Read the model definition and answer for the solid it produces. Units are mm, in the model's axes. Round coordinates to 2 decimals unless told otherwise and drop trailing zeros. Order: outer loops, then holes, each group sorted by start corner. A loop starts at its lowest first (then second) coordinate and runs counter-clockwise, first axis right, second up.
from build123d import *

# Parameters (mm, degrees)
SKETCH1_R      = 3
EXTRUDE4_DEPTH = 10
EXTRUDE5_DEPTH = 50


with BuildPart() as part:
    # Sketch1 → Extrude4 (new body)
    with BuildSketch(Plane.XY):
        with BuildLine():
            Line((-20, 13.266499161), (-20, -13.266499161))
            ThreePointArc((-20, -13.266499161), (0, -24), (20, -13.266499161))
            Line((20, -13.266499161), (20, 13.266499161))
            ThreePointArc((20, 13.266499161), (0, 24), (-20, 13.266499161))
        make_face()
        with BuildLine():
            ThreePointArc((-9.899494937, 9.899494937), (-5.357568053, 12.934313455), (0, 14))
            ThreePointArc((0, 14), (5.357568053, 12.934313455), (9.899494937, 9.899494937))
            ThreePointArc((9.899494937, 9.899494937), (14, 0), (9.899494937, -9.899494937))
            ThreePointArc((9.899494937, -9.899494937), (5.357568053, -12.934313455), (0, -14))
            ThreePointArc((0, -14), (-5.357568053, -12.934313455), (-9.899494937, -9.899494937))
            ThreePointArc((-9.899494937, -9.899494937), (-14, 0), (-9.899494937, 9.899494937))
        make_face(mode=Mode.SUBTRACT)
        with Locations((-13.435028843, 13.435028843)):
            Circle(SKETCH1_R, mode=Mode.SUBTRACT)
        with Locations((0, 19)):
            Circle(SKETCH1_R, mode=Mode.SUBTRACT)
        with Locations((13.435028843, 13.435028843)):
            Circle(SKETCH1_R, mode=Mode.SUBTRACT)
        with Locations((-13.435028843, -13.435028843)):
            Circle(SKETCH1_R, mode=Mode.SUBTRACT)
        with Locations((0, -19)):
            Circle(SKETCH1_R, mode=Mode.SUBTRACT)
        with Locations((13.435028843, -13.435028843)):
            Circle(SKETCH1_R, mode=Mode.SUBTRACT)
    extrude(amount=EXTRUDE4_DEPTH)

    # Sketch1<5> → Extrude5 (add)
    with BuildSketch(Plane.XY):
        with BuildLine():
            Line((0, 14), (0, 8))
            ThreePointArc((0, 8), (3.061467459, 7.39103626), (5.656854249, 5.656854249))
            Line((5.656854249, 5.656854249), (9.899494937, 9.899494937))
            ThreePointArc((9.899494937, 9.899494937), (5.357568053, 12.934313455), (0, 14))
        make_face()
        with BuildLine():
            ThreePointArc((-5.656854249, 5.656854249), (-3.061467459, 7.39103626), (0, 8))
            Line((0, 8), (0, 14))
            ThreePointArc((0, 14), (-5.357568053, 12.934313455), (-9.899494937, 9.899494937))
            Line((-9.899494937, 9.899494937), (-5.656854249, 5.656854249))
        make_face()
        with BuildLine():
            Line((9.899494937, 9.899494937), (5.656854249, 5.656854249))
            ThreePointArc((5.656854249, 5.656854249), (7.39103626, 3.061467459), (8, 0))
            Line((8, 0), (14, 0))
            ThreePointArc((14, 0), (12.934313455, 5.357568053), (9.899494937, 9.899494937))
        make_face()
        with BuildLine():
            ThreePointArc((8, 0), (7.39103626, -3.061467459), (5.656854249, -5.656854249))
            Line((5.656854249, -5.656854249), (9.899494937, -9.899494937))
            ThreePointArc((9.899494937, -9.899494937), (12.934313455, -5.357568053), (14, 0))
            Line((14, 0), (8, 0))
        make_face()
        with BuildLine():
            ThreePointArc((5.656854249, -5.656854249), (3.061467459, -7.39103626), (0, -8))
            Line((0, -8), (0, -14))
            ThreePointArc((0, -14), (5.357568053, -12.934313455), (9.899494937, -9.899494937))
            Line((9.899494937, -9.899494937), (5.656854249, -5.656854249))
        make_face()
        with BuildLine():
            Line((0, -14), (0, -8))
            ThreePointArc((0, -8), (-3.061467459, -7.39103626), (-5.656854249, -5.656854249))
            Line((-5.656854249, -5.656854249), (-9.899494937, -9.899494937))
            ThreePointArc((-9.899494937, -9.899494937), (-5.357568053, -12.934313455), (0, -14))
        make_face()
        with BuildLine():
            Line((-9.899494937, -9.899494937), (-5.656854249, -5.656854249))
            ThreePointArc((-5.656854249, -5.656854249), (-7.39103626, -3.061467459), (-8, 0))
            Line((-8, 0), (-14, 0))
            ThreePointArc((-14, 0), (-12.934313455, -5.357568053), (-9.899494937, -9.899494937))
        make_face()
        with BuildLine():
            ThreePointArc((-8, 0), (-7.39103626, 3.061467459), (-5.656854249, 5.656854249))
            Line((-5.656854249, 5.656854249), (-9.899494937, 9.899494937))
            ThreePointArc((-9.899494937, 9.899494937), (-12.934313455, 5.357568053), (-14, 0))
            Line((-14, 0), (-8, 0))
        make_face()
    extrude(amount=EXTRUDE5_DEPTH)


solid = part.part
Q1. Flat-ended cylindrical pins translate along their axes: pin 1 (1.5 mm diameter, centred on y = -4.5, z = 11, fed in from +X); pin 2 (1.5 mm diameter, centred on y = 2, z = 43.5, fed in from -X); pin 3 (12 mm diameter, centred on x = -5, z = 36.5, fed in from -Y). Find the tip coordinate at first contact, or state that the pin passes through.
Outcome:
pin 1: stops at x = 13.49
pin 2: stops at x = -13.94
pin 3: stops at y = -14
Q2. A cutting plane is placed at A-A, the plane z = 18.5. Give the vertices of the cut face in (x, y), plus the area to 3 significant figures.
Outcome:
outline: circle Ø28 at (0, 0); hole circle Ø16 at (0, 0)
area: 415 mm2
Q3. For a pull along Y with two mould halves and no side action, classify faces 1 (the face through (0, 24, 5)), 2 (the face through (-0.65, -21.93, 4.93)), 3 (the face through (-14, -5, 10)) as released by +Y, released by -Y, zero draft, split by the parting line, or undercut.
Outcome:
face 1: released by +Y
face 2: undercut
face 3: zero draft
Q4. A cutting plane is placed at C-C, the plane x = -15. Give the vertices of the cut face in (y, z) (1 decimal), plus the area to 3 significant figures.
Outcome:
outline: (-18.7, 0) - (-16, 0) - (-16, 10) - (-18.7, 10) - close; (-10.9, 0) - (10.9, 0) - (10.9, 10) - (-10.9, 10) - close; (16, 0) - (18.7, 0) - (18.7, 10) - (16, 10) - close
area: 272 mm2
Q5. A cutting plane is placed at D-D, the plane x = 12.5. Give the vertices of the cut face in (y, z).
Outcome:
outline: (-20.49, 0) - (-16.29, 0) - (-16.29, 10) - (-20.49, 10) - close; (-10.58, 0) - (10.58, 0) - (10.58, 10) - (6.3, 10) - (6.3, 50) - (-6.3, 50) - (-6.3, 10) - (-10.58, 10) - close; (16.29, 0) - (20.49, 0) - (20.49, 10) - (16.29, 10) - close
Q6. A cutting plane is placed at B-B, the plane y = -19. Give the vertices of the cut face in (x, z), plus the area to 3 significant figures.
Outcome:
outline: (-14.66, 0) - (-3, 0) - (-3, 10) - (-14.66, 10) - close; (3, 0) - (14.66, 0) - (14.66, 10) - (3, 10) - close
area: 233 mm2
Q7. Straight lines are drawn through the part: probe 1 along Y at (x, z) = (-14, 8.5); probe 2 along Z at (x, y) = (18.5, 13.5); probe 3 along X at (y, z) = (-15, 8) (1 decimal). For each, find the intervals that lie inside material, in ascending order.
Outcome:
probe 1: y = -19.49 to -16.38, -10.49 to 10.49, 16.38 to 19.49
probe 2: z = 0 to 10
probe 3: x = -18.7 to -16, -10.9 to 10.9, 16 to 18.7
